Autodesk Inventor part; units mm, degrees
ref_plane "YZ Plane" through (0, 0, 0) normal (1, 0, 0) x (0, 1, 0)
ref_plane "XZ Plane" through (0, 0, 0) normal (0, 1, 0) x (-1, 0, 0)
ref_plane "XY Plane" through (0, 0, 0) normal (0, 0, 1) x (1, 0, 0)
sketch "Sketch1" plane through (0, 0, 0) normal (0, 1, 0) x (-1, 0, 0)
  line L0 (105.8864, -9.1713) -> (29.6864, -9.1713)
  line L1 (29.6864, -9.1713) -> (29.6864, -59.9713)
  line L2 (29.6864, -59.9713) -> (105.8864, -59.9713)
  line L3 (105.8864, -59.9713) -> (105.8864, -9.1713)
  point P0 (0, 0)
  dimension "d0" = 76.2
  dimension "d1" = 50.8
extrude "Extrusion1" add sketch "Sketch1" along normal blind 16.51
sketch "Sketch2" plane through (0, 16.51, 0) normal (0, 1, 0) x (1, 0, 0)
  line L0 (-99.1001, 18.3012) -> (-96.0417, 26.9953) construction
  line L1 (-96.0417, 26.9953) -> (-92.1887, 31.3423) construction
  line L2 (-92.1887, 31.3423) -> (-84.285, 34.3061) construction
  line L3 (-84.285, 34.3061) -> (-80.6296, 29.3664) construction
  line L4 (-80.6296, 29.3664) -> (-77.2705, 18.3012) construction
  line L5 (-77.2705, 18.3012) -> (-76.579, 14.4191) construction
  spline S0 degree 4 poles (-99.1001, 18.3012) (-96.0417, 26.9953) (-92.1887, 31.3423) (-84.285, 34.3061) (-80.6296, 29.3664) (-77.2705, 18.3012) (-76.579, 14.4191) knots 1 1 1 1 1 2 3 4 4 4 4 4
  line L6 (-99.1001, 18.3012) -> (-99.1001, 25.8499) construction
  line L7 (-99.1001, 25.8499) -> (-96.5674, 31.3423) construction
  line L8 (-96.5674, 31.3423) -> (-93.9607, 34.9573) construction
  line L9 (-93.9607, 34.9573) -> (-88.2369, 37.0386) construction
  line L10 (-88.2369, 37.0386) -> (-83.2313, 37.9368) construction
  line L11 (-83.2313, 37.9368) -> (-75.6293, 34.8836) construction
  line L12 (-75.6293, 34.8836) -> (-71.3593, 29.3664) construction
  line L13 (-71.3593, 29.3664) -> (-68.785, 20.2226) construction
  line L14 (-68.785, 20.2226) -> (-68.785, 13.8588) construction
  spline S1 degree 4 poles (-99.1001, 18.3012) (-99.1001, 25.8499) (-96.5674, 31.3423) (-93.9607, 34.9573) (-88.2369, 37.0386) (-83.2313, 37.9368) (-75.6293, 34.8836) (-71.3593, 29.3664) (-68.785, 20.2226) (-68.785, 13.8588) knots 1 1 1 1 1 2 3 4 5 6 7 7 7 7 7
  line L15 (-68.2598, 29.584) -> (-66.503, 25.2471) construction
  line L16 (-66.503, 25.2471) -> (-65.2915, 22.9111) construction
  line L17 (-65.2915, 22.9111) -> (-65.2915, 14.27) construction
  spline S2 degree 3 poles (-68.2598, 29.584) (-66.503, 25.2471) (-65.2915, 22.9111) (-65.2915, 14.27) knots 1 1 1 1 2 2 2 2
  spline S3 degree 2 poles (-70.7555, 33.4961) (-73.1331, 37.1458) (-76.6265, 39.605) knots 0 0 0 1 1 1
  line L18 (-76.6265, 39.605) -> (-71.5951, 54.9343) construction
  line L19 (-71.5951, 54.9343) -> (-60.3667, 43.5663) construction
  line L20 (-60.3667, 43.5663) -> (-49.0964, 53.1455) construction
  spline S4 degree 3 poles (-76.6265, 39.605) (-71.5951, 54.9343) (-60.3667, 43.5663) (-49.0964, 53.1455) knots 1 1 1 1 2 2 2 2
  line L21 (-65.2915, 14.27) -> (-59.8318, 14.9374) construction
  line L22 (-59.8318, 14.9374) -> (-55.9104, 16.3841) construction
  line L23 (-55.9104, 16.3841) -> (-55.7779, 16.3841) construction
  spline S5 degree 3 poles (-65.2915, 14.27) (-59.8318, 14.9374) (-55.9104, 16.3841) (-55.7779, 16.3841) knots 1 1 1 1 2 2 2 2
  line L24 (-57.1115, 22.9111) -> (-55.7779, 16.3841) construction
  spline S6 degree 4 poles (-45.7217, 31.3084) (-51.5634, 33.293) (-56.0482, 30.8036) (-57.1115, 22.9111) (-55.7779, 16.3841) knots 1.168057 1.168057 1.168057 1.168057 1.168057 2 2 2 2 2
  line L25 (-45.7217, 31.3084) -> (-51.5634, 33.293) construction
  line L26 (-51.5634, 33.293) -> (-56.0482, 30.8036) construction
  line L27 (-56.0482, 30.8036) -> (-57.1115, 22.9111) construction
  line L28 (-45.7217, 31.3084) -> (-43.5479, 30.466) construction
  line L29 (-43.5479, 30.466) -> (-40.4918, 27.639) construction
  spline S7 degree 2 poles (-45.7217, 31.3084) (-43.5479, 30.466) (-40.4918, 27.639) knots 1 1 1 2 2 2
  line L30 (-40.4918, 27.639) -> (-44.1138, 33.293) construction
  line L31 (-44.1138, 33.293) -> (-48.4479, 36.0572) construction
  line L32 (-48.4479, 36.0572) -> (-52.5651, 39.1817) construction
  line L33 (-52.5651, 39.1817) -> (-59.6522, 37.2966) construction
  line L34 (-59.6522, 37.2966) -> (-64.7462, 34.8183) construction
  line L35 (-64.7462, 34.8183) -> (-68.2598, 29.584) construction
  spline S8 degree 4 poles (-40.4918, 27.639) (-44.1138, 33.293) (-48.4479, 36.0572) (-52.5651, 39.1817) (-59.6522, 37.2966) (-64.7462, 34.8183) (-68.2598, 29.584) knots 1 1 1 1 1 2 3 4 4 4 4 4
  spline S9 degree 4 poles (-70.7555, 33.4961) (-66.7607, 40.5932) (-58.5336, 42.023) (-54.7819, 41.9147) (-49.0964, 53.1455) knots 0 0 0 0 0 1 1 1 1 1
  line L36 (-76.579, 14.4191) -> (-73.1385, 13.5025) construction
  line L37 (-73.1385, 13.5025) -> (-68.785, 13.8588) construction
  spline S10 degree 2 poles (-76.579, 14.4191) (-73.1385, 13.5025) (-68.785, 13.8588) knots 1 1 1 2 2 2
  point P0 (0, 0)
  point P1 (-73.4266, 36.8633)
  point P2 (-65.6468, 38.768)
  point P3 (-60.3715, 41.5372)
  point P4 (-55.5489, 44.3879)
sketch "Sketch5" plane through (0, 16.51, 0) normal (0, 1, 0) x (1, 0, 0)
  circle A0 centre (-39.7111, 26.2451) radius 1.5875
  circle A1 centre (-99.3276, 16.7185) radius 1.5875
  circle A2 centre (-48.3267, 54.5366) radius 1.5875
  point P0 (0, 0)
extrude "Extrusion8" add sketch "Sketch2" along normal blind 2.54
extrude "Extrusion9" cut sketch "Sketch5" against normal blind 2.54
properties part number "cimproj"
Input: part model. Units: mm. Frame: model coordinates. A direction names the side the tool comes from. Coordinates: 2 decimals unless noted, no trailing zeros. Loops run counter-clockwise (first coordinate to the right, second up) from the corner with the lowest first, then second, coordinate; pieces in that order, holes last. Notation, with made-up numbers: (75, 34.5) -> (114, 34.5) arc R25 cw to (114, 56.5) -> close; hole circle Ø5 at (86.5, 63.25). An arc over 180 degrees is marked (long way). Write each question's results on one line, items separated by ' | '. Start each with the question number.
Q1. Pull-direction query (X, two-part tool) for faces 1 (the flat face through (-40, 13.97, -26)), 2 (the flat face through (-29.686, 8, -34)), 3 (the flat face through (-67, 0, -34)); classes: released by +X, released by -X, zero draft, split by the parting line, or undercut.
Q2. Ray query, line 1 (Y direction, x = -48, z = -20.5); line 2 (Y direction, x = -39.5, z = -25); line 3 (Z direction, x = -47, y = 15). Return the intervals inside material, ascending. Write a range as from..to.
Q3. Reachability of faces 4 (the flat face through (-81, 19.05, -29)), 5 (the cylindrical face through (-97.86, 15.26, -16.11)) from +Z, -Z, +X, -X, +Y, -Y: full face, straight path, thin tool, end or side. Return the list, or none.
Q4. Pin query (flat end, axial travel): pin 1 (2 mm diameter, centred on x = -61, z = -22, fed in from -Y); pin 2 (3.5 mm diameter, centred on x = -100, z = -16.5, fed in from +Y); pin 3 (1 mm diameter, centred on x = -39.5, z = -26.5, fed in from +Y). Return the tip coordinate at first contact, or that it passes through.
Q5. Section A-A, the plane x = -39. Return the cut outline in (y, z).
Found:
1) face 1: undercut | face 2: released by +X | face 3: zero draft
2) line 1: 0..16.51 | line 2: 0..13.97 | line 3: -59.97..-55.41, -53.66..-9.17
3) face 4: +Z, -Z, +X, -X, +Y | face 5: +Y
4) pin 1: y = 0 | pin 2: y = 16.51 | pin 3: y = 13.97
5) outline: (0, -59.97) -> (16.51, -59.97) -> (16.51, -27.66) -> (13.97, -27.66) -> (13.97, -24.83) -> (16.51, -24.83) -> (16.51, -9.17) -> (0, -9.17) -> close
